For this review, take the finished solid that the model builds, in its own axes (mm). A direction names the side the tool comes from. Round coordinates to 2 decimals unless told otherwise and drop trailing zeros. Write each loop counter-clockwise with the first axis right and the second up, starting at its lowest first coordinate (ties: lowest second). Pieces come first, ordered by that corner, then holes. Notation, with made-up numbers: M 7.5,40.25 L 40.5,40.25 A27 cw 40.5,68.25 Z; hole C 11,-29 d6. An arc over 180 degrees is marked long. Use one line per item in the form item = value. Start each with the question number.
Item 1: For faces 1 (the cylindrical face through (2.703, 2.958, 8.584)), 2 (the flat face through (-6, 6, 2)), list the 3-axis set-ups (+Z, -Z, +X, -X, +Y, -Y) from which the entire face can be reached by the end or side of a thin tool; tool diameter is ignored.
Item 2: Add section C-C (y = 4.5). State the section outline as (x, z) points.
Item 3: Add section A-A (z = 0). State the section outline as (x, y) points.
Item 4: Add section D-D (y = 6.25). State the section outline as (x, z) points, and give its area (3 significant figures).
Item 5: Add section B-B (x = 0). State the section outline as (y, z) points, and give its area (3 significant figures).
Item 6: For P1, Ø1, axis at x = -6, z = -2.5, coming from the +Y side; P2, Ø6, axis at x = -4, y = 6.5, coming from the -Z side; P3, Ø6, axis at x = -5, y = 7.5, coming from the +Z side, all flat-tipped, find the tip position at first contact; note any pin that passes through.
Item 7: For line 1 (Y direction, x = -5, z = -6.5); line 2 (Z direction, x = 2.5, y = 10); line 3 (X direction, y = 2, z = 1.5), list the stretches that pass through material, from the lowest coordinate up. Write a range as [from, to].
from build123d import *

# Parameters (mm, degrees)
SKETCH1_R           = 9
BOSS_EXTRUDE1_DEPTH = 6
SKETCH2_R           = 5.9
BOSS_EXTRUDE2_DEPTH = 20
SKETCH5_R           = 9.837832021
CUT_EXTRUDE3_DEPTH  = 14.1


with BuildPart() as part:
    # Sketch1 → Boss-Extrude1 (new body)
    with BuildSketch(Plane(origin=(0, 0, 0), x_dir=(1, 0, 0), z_dir=(0, 1, 0))):
        with Locations(Location((0, 0, 0), (0, 0, 270))):
            Circle(SKETCH1_R)
    extrude(amount=BOSS_EXTRUDE1_DEPTH)

    # Sketch2 → Boss-Extrude2 (add)
    with BuildSketch(Plane(origin=(0, 6, 0), x_dir=(1, 0, 0), z_dir=(0, 1, 0))):
        with Locations(Location((0, 0, 0), (0, 0, 270))):
            Circle(SKETCH2_R)
    extrude(amount=BOSS_EXTRUDE2_DEPTH)

    # Sketch5 → Cut-Extrude3 (cut)
    with BuildSketch(Plane(origin=(0, 26, 0), x_dir=(1, 0, 0), z_dir=(0, 1, 0))):
        Circle(SKETCH5_R)
    extrude(amount=-CUT_EXTRUDE3_DEPTH, mode=Mode.SUBTRACT)


solid = part.part
Calculated:
q1.face_1 = +Y, -Y
q1.face_2 = +Y
q2.outline = C 0,0 d18
q3.outline = M -9,0 L 9,0 L 9,6 L 5.9,6 L 5.9,11.9 L -5.9,11.9 L -5.9,6 L -9,6 Z
q4.outline = C 0,0 d11.8
q4.area = 109 mm^2
q5.outline = M 0,-9 L 6,-9 L 6,-5.9 L 11.9,-5.9 L 11.9,5.9 L 6,5.9 L 6,9 L 0,9 Z
q5.area = 178 mm^2
q6.P1 = 6
q6.P2 = -8.94
q6.P3 = 8.67
q7.line_1 = [0, 6]
q7.line_2 = [-5.34, 5.34]
q7.line_3 = [-8.87, 8.87]
